Could you check a few things on this model? Use its own coordinates, in mm. Face numbers are marked on the shaded views. A direction names the side the tool comes from. Give positions to 0.01 mm unless a question says otherwise; leave off trailing zeros. Order: outer loops, then holes, each group sorted by start corner. A loop starts at its lowest first (then second) coordinate and runs counter-clockwise, first axis right, second up. Notation, with made-up numbers: M 71.25,-21.5 L 84.25,-21.5 A23 cw 84.25,10.5 Z; hole C 59.5,35.5 d2. An arc over 180 degrees is marked long. Use a Markdown table: item, result. Add a question column.
Item 1: I'm going to push flat-ended pins straight in: pin 1 Ø5 at (x, z) = (5.5, 25.5) entering from -Y; pin 2 Ø1.5 at (x, z) = (-0.5, 13.5) entering from +Y; pin 3 Ø10 at (x, y) = (0, 0) entering from +Z; pin 4 Ø4 at (x, z) = (8.5, 9) entering from +Y. Where does each tip first touch, or does it pass through?
Item 2: If I drill on L1, parallel to Y at x = 0, z = 75.5; L2, parallel to X at y = 13, z = 62.5; L3, parallel to Z at x = -1, y = 21.5, over which ranges is the centre line in solid material (lowest first)? Write a range as from..to.
Item 3: Suppose I cut it at C-C on z = 52. Write out the boundary of the cut face in (x, y), plus the area to 3 significant figures.
Item 4: Suppose I cut it at A-A on x = 0. Write out the boundary of the cut face in (y, z).
Item 5: Suppose I cut it at B-B on z = -25.5. Write out the boundary of the cut face in (x, y).
Item 6: For the marked faces 1, 2, 3, 4 and 5, which set-ups out of +Z, -Z, +X, -X, +Y, -Y let a thin tool reach every point of the face, with its end or its side?
from build123d import *

# Parameters (mm, degrees)
SKETCH1_R           = 15
BOSS_EXTRUDE1_DEPTH = 80
SKETCH1_2_R         = 15
SKETCH2_R           = 25
SKETCH3_R           = 7.5
BOSS_EXTRUDE2_DEPTH = 25
SKETCH4_W           = 5
SKETCH4_H           = 25
BOSS_EXTRUDE3_DEPTH = 10
SKETCH5_R           = 3.15
CUT_EXTRUDE1_DEPTH  = 6
SKETCH6_R           = 20
BOSS_EXTRUDE4_DEPTH = 15


with BuildPart() as part:
    # Sketch1 → Boss-Extrude1 (new body)
    with BuildSketch(Plane.XY):
        Circle(SKETCH1_R)
    extrude(amount=BOSS_EXTRUDE1_DEPTH)

    # Sketch1<2> → Loft1 section 0
    with BuildSketch(Plane.XY):
        Circle(SKETCH1_2_R)
    # Sketch2 → Loft1 section 1
    with BuildSketch(Plane(origin=(0, 0, -10), x_dir=(-1, 0, 0), z_dir=(0, 0, -1))):
        Circle(SKETCH2_R)
    loft()

    # Sketch3 → Boss-Extrude2 (add)
    with BuildSketch(Plane(origin=(0, 0, -10), x_dir=(-1, 0, 0), z_dir=(0, 0, -1))):
        Circle(SKETCH3_R)
    extrude(amount=BOSS_EXTRUDE2_DEPTH)

    # Sketch4 → Boss-Extrude3 (add)
    with BuildSketch(Plane.XY.offset(10)):
        with Locations((0.003158662, 12.374368268)):
            Rectangle(SKETCH4_W, SKETCH4_H)
    extrude(amount=BOSS_EXTRUDE3_DEPTH)

    # Sketch5 → Cut-Extrude1 (cut)
    with BuildSketch(Plane.XY.offset(80)):
        Circle(SKETCH5_R)
    extrude(amount=-CUT_EXTRUDE1_DEPTH, mode=Mode.SUBTRACT)

    # Sketch6 → Boss-Extrude4 (add)
    with BuildSketch(Plane.XY.offset(10)):
        Circle(SKETCH6_R)
    extrude(amount=-BOSS_EXTRUDE4_DEPTH)


solid = part.part
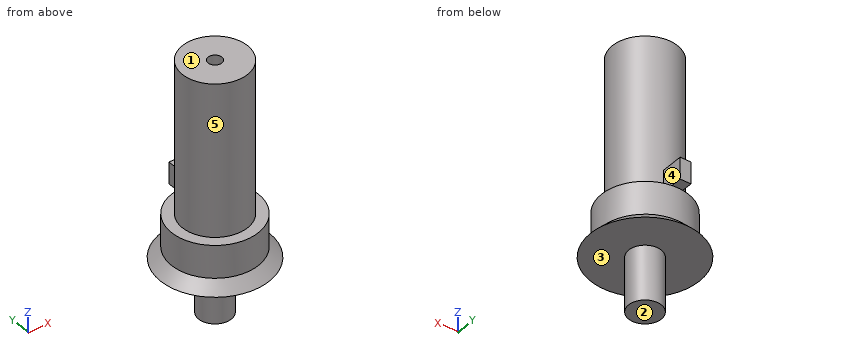
Findings below:
| question | item | result |
|---|---|---|
| 1 | pin 1 | stops at y = -14.7 |
| 1 | pin 2 | stops at y = 24.87 |
| 1 | pin 3 | stops at z = 80 |
| 1 | pin 4 | stops at y = 18.91 |
| 2 | L1 | y = -15..-3.15, 3.15..15 |
| 2 | L2 | x = -7.48..7.48 |
| 2 | L3 | z = -10..-6.52, 10..20 |
| 3 | outline | C 0,0 d30 |
| 3 | area | 707 mm^2 |
| 4 | outline | M -25,-10 L -7.5,-10 L -7.5,-35 L 7.5,-35 L 7.5,-10 L 25,-10 L 20,-5 L 20,10 L 24.87,10 L 24.87,20 L 15,20 L 15,80 L 3.15,80 L 3.15,74 L -3.15,74 L -3.15,80 L -15,80 L -15,10 L -20,10 L -20,-5 Z |
| 5 | outline | C 0,0 d15 |
| 6 | face 1 | +Z, +X, -X, +Y, -Y |
| 6 | face 2 | -Z, +X, -X, +Y, -Y |
| 6 | face 3 | -Z |
| 6 | face 4 | +Z, +X, +Y |
| 6 | face 5 | +Z |
